Here's how the part is built. I have some questions about the finished solid (model axes, mm). A direction names the side the tool comes from. Round coordinates to 2 decimals unless told otherwise and drop trailing zeros. Write each loop counter-clockwise with the first axis right and the second up, starting at its lowest first coordinate (ties: lowest second). Pieces come first, ordered by that corner, then holes. Notation, with made-up numbers: (78, 79) -> (82, 79) arc R5 ccw to (82, 84) -> close; hole circle Ø8 at (-3, -1.75). An arc over 180 degrees is marked (long way). Put each result on its own line as item: value. Start each with the question number.
1) I want a section at D-D, the plane z = 10. List the corners of the cut face in (x, y) for me.
2) Which directions (+Z, -Z, +X, -X, +Y, -Y) give clear straight access to the entire face, cutting with the end or side of a thin tool? Please do faces 1 (the flat face through (4.5, 19, 0)), 2 (the cylindrical face through (6.215, 19.703, -6.199)), 3 (the flat face through (0, 19, 6.5)), 4 (the cylindrical face through (-6.199, 19.703, 6.215)).
3) If I drill on line 1 along X through (y, z) = (1, 0); line 2 along Z through (x, y) = (1, 14), over which ranges is the centre line in solid material (lowest first)? Write a range as [from, to].
4) I want a section at B-B, the plane y = 9. List the corners of the cut face in (x, z) for me.
5) We'd pull the mould along X, two halves only. Please class faces 5 (the cylindrical face through (-3.593, 2.465, 1.869)), 6 (the flat face through (-8, 5, 0)), 7 (the cylindrical face through (6.199, 19.703, 6.215)), 8 (the cylindrical face through (0.07, 2.46, -11.5)): released by +X, released by -X, zero draft, split by the parting line, or undercut.
6) Will these pins go through, and if not, where does the flat tip stop? P1, Ø2.5, axis at x = -1, z = -1.5, coming from the +Y side; P2, Ø1.5, axis at x = 11, z = 0, coming from the +Y side; P3, Ø9, axis at y = 13, z = 2, coming from the +X side; P4, Ø10, axis at x = 2.5, y = 10.5, coming from the +Z side.
7) I want a section at A-A, the plane z = 0. Give the number of separate pieces and of enclosed holes in the cut face, then the cut area to 3 significant figures.
from build123d import *

# Parameters (mm, degrees)
SKETCH_1_R      = 17.5
SKETCH_1_R_2    = 4.05
SKETCH_1_R_3    = 1.5
EXTRUDE_1_DEPTH = 5
SKETCH_2_W      = 13
SKETCH_2_H      = 13
SKETCH_2_W_2    = 9
SKETCH_2_H_2    = 9
EXTRUDE_2_DEPTH = 30
FILLET_1_R      = 1


with BuildPart() as part:
    # 草图1 → 凸台-拉伸1 (new body)
    with BuildSketch(Plane(origin=(0, 0, 0), x_dir=(1, 0, 0), z_dir=(0, 1, 0))):
        with Locations(Location((0, 0, 0), (0, 0, 270))):
            Circle(SKETCH_1_R)
        with Locations(Location((0, 0, 0), (0, 0, 270))):
            Circle(SKETCH_1_R_2, mode=Mode.SUBTRACT)
        with Locations(Location((0, 10, 0), (0, 0, 270))):
            Circle(SKETCH_1_R_3, mode=Mode.SUBTRACT)
        with Locations(Location((10, 0, 0), (0, 0, 270))):
            Circle(SKETCH_1_R_3, mode=Mode.SUBTRACT)
        with Locations(Location((0, -10, 0), (0, 0, 270))):
            Circle(SKETCH_1_R_3, mode=Mode.SUBTRACT)
        with Locations(Location((-10, 0, 0), (0, 0, 270))):
            Circle(SKETCH_1_R_3, mode=Mode.SUBTRACT)
    extrude(amount=EXTRUDE_1_DEPTH)

    # 草图2 → 凸台-拉伸2 (add)
    with BuildSketch(Plane(origin=(0, 5, 0), x_dir=(1, 0, 0), z_dir=(0, 1, 0))):
        Rectangle(SKETCH_2_W, SKETCH_2_H)
        Rectangle(SKETCH_2_W_2, SKETCH_2_H_2, mode=Mode.SUBTRACT)
    extrude(amount=EXTRUDE_2_DEPTH)

    # 圆角1
    fillet_1_edges = [part.edges().sort_by_distance(p)[0] for p in [
        (0, 35, -6.5),
        (-6.5, 35, 0),
        (0, 35, 6.5),
        (6.5, 35, 0),
        (6.5, 20, -6.5),
        (-6.5, 20, -6.5),
        (-6.5, 20, 6.5),
        (6.5, 20, 6.5),
        (-4.5, 35, 0),
        (0, 35, 4.5),
        (4.5, 35, 0),
        (0, 35, -4.5),
    ]]
    fillet(fillet_1_edges, radius=FILLET_1_R - 0.0001)  # a hair under: the kernel refuses the full size


solid = part.part
Findings:
1. outline: (-14.36, 0) -> (-1.5, 0) -> (-1.5, 5) -> (-14.36, 5) -> close; (1.5, 0) -> (14.36, 0) -> (14.36, 5) -> (1.5, 5) -> close
2. face 1: +Y
2. face 2: -Z, +X, +Y
2. face 3: +Z, +X, -X, +Y
2. face 4: +Z, -X, +Y
3. line 1: x = [-17.5, -11.5], [-8.5, -4.05], [4.05, 8.5], [11.5, 17.5]
3. line 2: z = [-6.5, -4.5], [4.5, 6.5]
4. outline: (-6.5, -5.5) arc R1 ccw to (-5.5, -6.5) -> (5.5, -6.5) arc R1 ccw to (6.5, -5.5) -> (6.5, 5.5) arc R1 ccw to (5.5, 6.5) -> (-5.5, 6.5) arc R1 ccw to (-6.5, 5.5) -> close; hole (-4.5, -4.5) -> (4.5, -4.5) -> (4.5, 4.5) -> (-4.5, 4.5) -> close
5. face 5: undercut
5. face 6: zero draft
5. face 7: released by +X
5. face 8: undercut
6. P1: passes through
6. P2: stops at y = 5
6. P3: stops at x = 6.5
6. P4: stops at z = 6.5
7. separate pieces: 4
7. enclosed holes: 0
7. area: 224 mm2
